Geometry: see drawing. Coordinates: mm, zero at the bounding-box minimum. Round coordinates to 2 decimals unless told otherwise and drop trailing zeros. Write each loop counter-clockwise with the first axis right and the second up, starting at its lowest first coordinate (ties: lowest second). Pieces come first, ordered by that corner, then holes. Notation, with made-up numbers: (48, 34.5) -> (88, 34.5) arc R26 cw to (88, 56.5) -> close; hole circle Ø11 at (-17.75, 54.5). An arc over 180 degrees is marked (long way). Use CSV: the item, a comma, the result in double quotes.
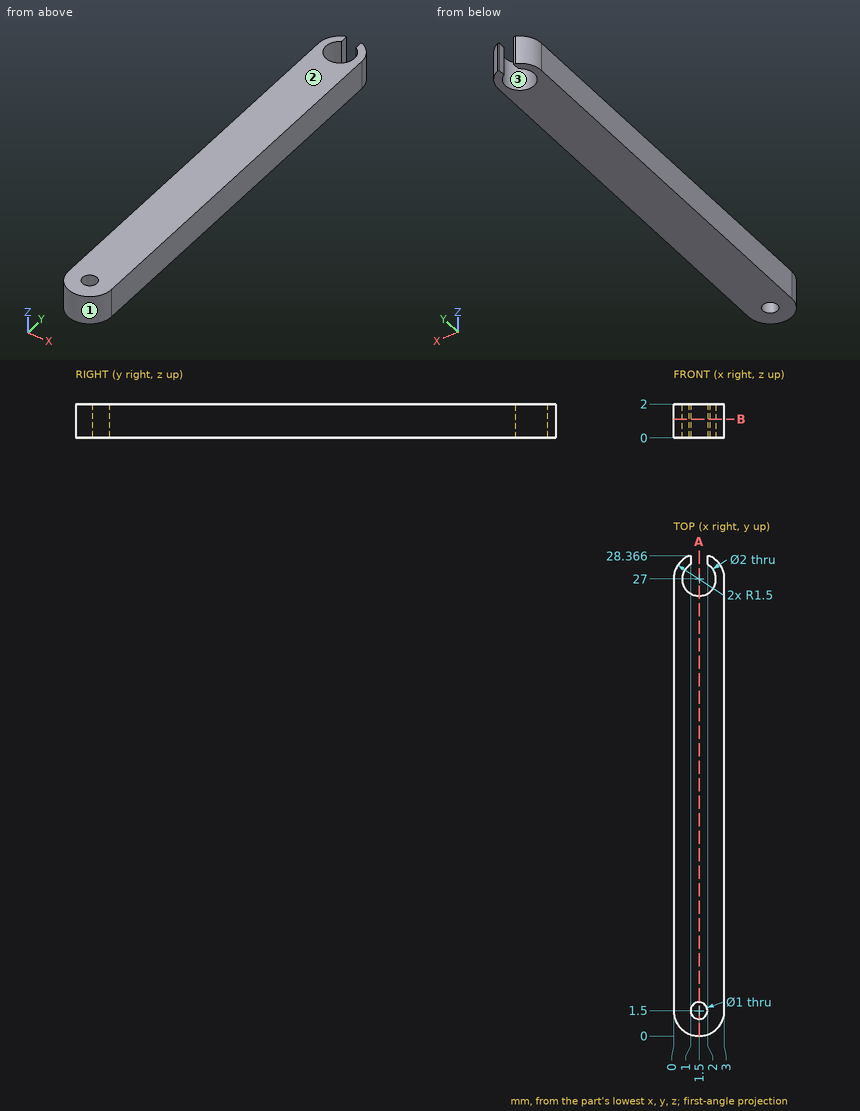
Item 1: Line query: line 1 (Y direction, x = 1.5, z = 1); line 2 (Y direction, x = 1.2, z = 1.4); line 3 (X direction, y = 1.75, z = 1.65). Output: solid intervals per line, ascending.
Worked answers:
line 1,"y = 0 to 1, 2 to 26"
line 2,"y = 0.03 to 1.1, 1.9 to 26.05"
line 3,"x = 0 to 1.07, 1.93 to 3"
Item 2: Section query A-A on x = 1.5. Return the cut outline in (y, z), plus the area to 3 significant figures.
Worked answers:
outline,"(0, 0) -> (1, 0) -> (1, 2) -> (0, 2) -> close; (2, 0) -> (26, 0) -> (26, 2) -> (2, 2) -> close"
area,"50.0 mm²"
Item 3: Pull-direction query (Y, two-part tool) for the marked faces 1, 2 and 3; classes: +Y half, -Y half, draft (parallel to the pull), parting line (faces both ways), or undercut.
Worked answers:
face 1,"-Y half"
face 2,"draft"
face 3,"undercut"
Item 4: First-contact query: pin 1 Ø0.6 at (y, z) = (28, 1.5) entering from -X; pin 2 Ø1.2 at (x, y) = (1.5, 27) entering from +Z. Flat tips, straight axial feed; report the tip coordinate or a pass-through.
Worked answers:
pin 1,"stops at x = 0.17"
pin 2,"passes through"
Item 5: Section query B-B on z = 1.1. Return the cut outline in (x, y).
Worked answers:
outline,"(0, 1.5) arc R1.5 ccw to (3, 1.5) -> (3, 27) arc R1.5 ccw to (2.12, 28.37) -> (2, 28.37) -> (2, 27.87) arc R1 cw (long way) to (1, 27.87) -> (1, 28.37) -> (0.88, 28.37) arc R1.5 ccw to (0, 27) -> close; hole circle Ø1 at (1.5, 1.5)"
